```python
from build123d import *

# Parameters (mm, degrees)
F1_DEPTH = 101.6
F2_W     = 50.8
F2_H     = 38.1
F3_DEPTH = 19.05


with BuildPart() as f1:
    # F0 (on Front) → F1 (new body)
    with BuildSketch(Plane.XZ):
        Polygon((-29.8929, -17.777541), (-29.8929, -43.177541), (33.6071, -43.177541), (33.6071, 33.022459), (-4.4929, 33.022459), (-4.4929, -17.777541), align=None)
    extrude(amount=F1_DEPTH)

    # F2 (on face) → F3 (cut)
    with BuildSketch(Plane(origin=(-4.4929, 0, 0), x_dir=(0, -1, 0), z_dir=(-1, 0, 0))):
        with Locations((50.8, 13.972459)):
            Rectangle(F2_W, F2_H)
    extrude(amount=-F3_DEPTH, mode=Mode.SUBTRACT)


solid = f1.part
```
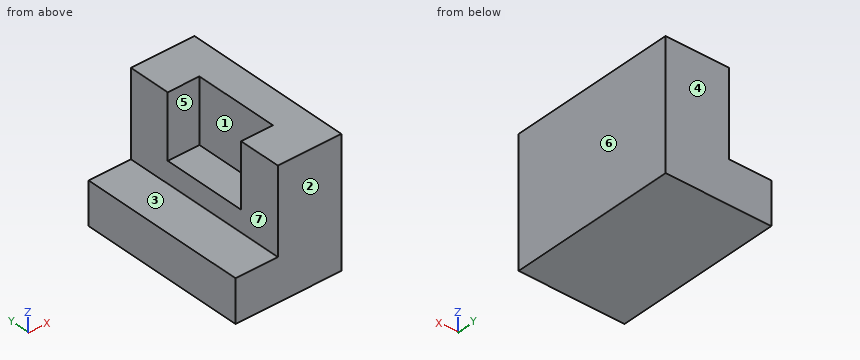
Could you check a few things on this model? Use its own coordinates, in mm. Face numbers are marked on the shaded views. A direction names the side the tool comes from. Give positions to 0.01 mm unless a question says otherwise; leave off trailing zeros. Order: outer loops, then holes, each group sorted by start corner. A loop starts at its lowest first (then second) coordinate and runs counter-clockwise, first axis right, second up.
Q1. For the marked faces 5, 6 and 7, which set-ups out of +Z, -Z, +X, -X, +Y, -Y let a thin tool reach every point of the face, with its end or its side?
Q2. Suppose I cut it at D-D, the plane y = -21. Write out the boundary of the cut face in (x, z).
Q3. Suppose I cut it at B-B, the plane z = 0. Write out the boundary of the cut face in (x, y), and give its area (3 significant figures).
Q4. We'd pull the mould along Y, two halves only. Please class the marked faces 1, 2, 3 and 4: +Y half, -Y half, draft (parallel to the pull), parting line (faces both ways), or undercut.
Q5. If I drill on line 1 along Y through (x, z) = (3, 1); line 2 along X through (y, z) = (-12, 5.5); line 3 along Z through (x, y) = (-4, -45.5), over which ranges is the centre line in solid material (lowest first)?
Q6. Suppose I cut it at C-C, the plane x = -22. Write out the boundary of the cut face in (y, z), and give its area (3 significant figures).
Q7. I'm going to push flat-ended pins straight in: P1, Ø9.5, axis at x = 5.5, z = 8, coming from the +Y side; P2, Ø9.5, axis at x = 6.5, y = -41, coming from the +Z side; P3, Ø20.5, axis at x = -19.5, y = -38.5, coming from the +Z side; P4, Ø1, axis at y = -14.5, z = 6.5, coming from the -X side. Where does each tip first touch, or does it pass through?
Q8. Suppose I cut it at A-A, the plane y = -35.5. Write out the boundary of the cut face in (x, z), and give its area (3 significant figures).
Solution:
1. face 5: +Z, -X
1. face 6: +Z, -Z, +X, +Y, -Y
1. face 7: +Z, -X, +Y, -Y
2. outline: (-29.89, -43.18) - (33.61, -43.18) - (33.61, 33.02) - (-4.49, 33.02) - (-4.49, -17.78) - (-29.89, -17.78) - close
3. outline: (-4.49, -101.6) - (33.61, -101.6) - (33.61, 0) - (-4.49, 0) - (-4.49, -25.4) - (14.56, -25.4) - (14.56, -76.2) - (-4.49, -76.2) - close
3. area: 2,900 mm2
4. face 1: undercut
4. face 2: -Y half
4. face 3: draft
4. face 4: +Y half
5. line 1: y = -101.6 to -76.2, -25.4 to 0
5. line 2: x = -4.49 to 33.61
5. line 3: z = -43.18 to -5.08
6. outline: (-101.6, -43.18) - (0, -43.18) - (0, -17.78) - (-101.6, -17.78) - close
6. area: 2,580 mm2
7. P1: stops at y = 0
7. P2: stops at z = -5.08
7. P3: stops at z = -17.78
7. P4: stops at x = -4.49
8. outline: (-29.89, -43.18) - (33.61, -43.18) - (33.61, 33.02) - (14.56, 33.02) - (14.56, -5.08) - (-4.49, -5.08) - (-4.49, -17.78) - (-29.89, -17.78) - close
8. area: 2,820 mm2
